```python
from build123d import *

# Parameters (mm, degrees)
EXTRUDE_1_DEPTH     = 6
EXTRUDE_2_DEPTH     = 4.2
SKETCH_3_R          = 2.35
EXTRUDE_3_DEPTH     = 2.8
SWEEP_START         = -2
SWEEP_1_DEPTH       = 4
CUT_EXTRUDE_1_DEPTH = 3


# Read off the part's stored shape, not the designer's step: По траектории1
with BuildPart() as part:
    # Эскиз1 → Бобышка-Вытянуть1 (new, symmetric)
    with BuildSketch(Plane(origin=(0, 0, 0), x_dir=(0, 0, -1), z_dir=(1, 0, 0))):
        Polygon((0, 0), (22, 0), (22, 19.3), (27, 19.3), (27, 21.8), (22, 21.8), (22, 26), (0, 26), (0, 21.8), (-5, 21.8), (-5, 19.3), (0, 19.3), align=None)
    extrude(amount=EXTRUDE_1_DEPTH, both=True)

    # Эскиз2 → Бобышка-Вытянуть2 (add)
    with BuildSketch(Plane(origin=(0, 26, 0), x_dir=(1, 0, 0), z_dir=(0, 1, 0))):
        with BuildLine():
            Line((-2.75, 12), (-2.75, 11.332682252))
            ThreePointArc((-2.75, 11.332682252), (0, 0), (2.75, 11.332682252))
            Line((2.75, 11.332682252), (2.75, 12))
            ThreePointArc((2.75, 12), (0, 14.75), (-2.75, 12))
        make_face()
    extrude(amount=EXTRUDE_2_DEPTH)

    # Эскиз3 → Бобышка-Вытянуть3 (add)
    with BuildSketch(Plane(origin=(0, 30.2, 0), x_dir=(1, 0, 0), z_dir=(0, 1, 0))):
        with Locations(Location((0, 6, 0), (0, 0, 270))):
            Circle(SKETCH_3_R)
    extrude(amount=EXTRUDE_3_DEPTH)

    # По траектории1 outline → По траектории1 (add)
    with BuildSketch(Plane.YZ.offset(SWEEP_START)):
        with BuildLine():
            Line((7.5, -22), (5, -22))
            add(Edge.make_bspline(
                [(5, -22), (5.069741994, -22.788251561), (5.125958635, -24.404153677), (4.878573381, -26.772120173), (4.395772619, -28.378294328), (3.83166606, -29.588406839), (3.21879889, -30.61604033), (2.403361035, -31.959681467), (1.936450048, -33.447187834), (1.879246473, -34.586937516), (2.09656871, -35.628227488), (2.472597261, -36.523725644), (2.84782964, -37.107918611), (3.067609014, -37.407797225)],
                knots=[0, 0, 0, 0, 0.166666667, 0.333333333, 0.5, 0.534253468, 0.625, 0.75, 0.8125, 0.875, 0.916666667, 0.958333333, 1, 1, 1, 1], degree=3))
            Line((3.067609014, -37.407797225), (5.173227765, -36.060069628))
            add(Edge.make_bspline(
                [(7.5, -22), (7.567173372, -22.882492449), (7.618252767, -24.686876341), (7.299304344, -27.455245749), (6.663696491, -29.460064755), (5.924563706, -30.955136787), (5.18985295, -32.152025941), (4.582294135, -33.24339685), (4.389602767, -34.062522123), (4.406362916, -34.546823904), (4.535371286, -35.013924669), (4.759350216, -35.482390845), (5.013826459, -35.862321947), (5.173227765, -36.060069628)],
                knots=[0, 0, 0, 0, 0.166666667, 0.333333333, 0.5, 0.534253468, 0.625, 0.75, 0.8125, 0.875, 0.916666667, 0.958333333, 1, 1, 1, 1], degree=3))
        make_face()
    extrude(amount=SWEEP_1_DEPTH)

    # Эскиз6 → Вырез-Вытянуть1 (cut)
    with BuildSketch(Plane(origin=(0, 21.8, 0), x_dir=(1, 0, 0), z_dir=(0, 1, 0))):
        with BuildLine():
            Line((-0.5, 27), (-0.5, 25.645643924))
            ThreePointArc((-0.5, 25.645643924), (0, 23.25), (0.5, 25.645643924))
            Line((0.5, 25.645643924), (0.5, 27))
            Line((0.5, 27), (0, 27))
            Line((0, 27), (-0.5, 27))
        make_face()
        with BuildLine():
            Line((0.5, -5), (0.5, -3.645643924))
            ThreePointArc((0.5, -3.645643924), (0, -1.25), (-0.5, -3.645643924))
            Line((-0.5, -3.645643924), (-0.5, -5))
            Line((-0.5, -5), (0, -5))
            Line((0, -5), (0.5, -5))
        make_face()
    extrude(amount=-CUT_EXTRUDE_1_DEPTH, mode=Mode.SUBTRACT)


solid = part.part
```
Part model, mm, in its own coordinate system. A direction names the side the tool comes from. Give positions to 0.01 mm unless a question says otherwise; leave off trailing zeros. Write each loop counter-clockwise with the first axis right and the second up, starting at its lowest first coordinate (ties: lowest second). Pieces come first, ordered by that corner, then holes. Notation, with made-up numbers: (13, -33) -> (20, -33) arc R9 cw to (20, -26) -> close; hole circle Ø6 at (21.5, 60). An arc over 180 degrees is marked (long way). Put each result on its own line as item: value. Start each with the question number.
Item 1: Cut at C-C (z = -24.5). State how many separate pieces and enclosed holes the cut face has, then the cut area to 3 significant figures.
Item 2: Which spindle directions (+Z, -Z, +X, -X, +Y, -Y) get a long thin tool onto all of the face, cutting with end or side? Do faces 5 (the face through (-0.5, 21, 4)), 6 (the face through (1.42, 21.8, -24.54)), 7 (the face through (1.42, 21.8, 2.47)). Say none if no direction does.
Item 3: Cut at A-A (z = 2.5). List the corners of the cut face in (x, y), then the cut area to 4 significant figures.
Item 4: Cut at D-D (y = 17.5). List the corners of the cut face in (x, z), then the cut area to 3 significant figures.
Item 5: Wall check: L1, parallel to X at y = 20.15, z = -24.5; L2, parallel to Y at x = 5.25, z = -2; L3, parallel to Y at x = 3, z = 1.5. Give the ranges that are in metal, low to high. Write a range as [from, to].
Item 6: Cut at B-B (x = -4.25). List the corners of the cut face in (y, z).
Item 7: Pin check, flat tips, straight feed: pin 1 Ø3 at (x, z) = (-1.5, -2) entering from +Y; pin 2 Ø3 at (x, z) = (-1, -31.5) entering from +Y; pin 3 Ø5.5 at (x, z) = (-2, -23.5) entering from +Y. Stop position of each tip, or through.
Item 8: Pull direction X, two halves, no side cores. Call faces 1 (the face through (0, 26, -16)), 2 (the face through (2, 5, -30)), 3 (the face through (0.06, 28.07, -14.75)), 4 (the face through (-0.05, 20.57, -23.25)): pulls with the +X half, pulls with the -X half, needs draft (parallel to the pull), parting line crosses it, or undercut.
Answer list:
1. separate pieces: 3
1. enclosed holes: 0
1. area: 33.7 mm2
2. face 5: +Z, +Y, -Y
2. face 6: -Z, +X, -X, +Y
2. face 7: +Z, +X, -X, +Y
3. outline: (-6, 19.3) -> (-1.25, 19.3) -> (-1.25, 21.8) -> (-6, 21.8) -> close; (1.25, 19.3) -> (6, 19.3) -> (6, 21.8) -> (1.25, 21.8) -> close
3. area: 23.75 mm2
4. outline: (-6, -22) -> (6, -22) -> (6, 0) -> (-6, 0) -> close
4. area: 264 mm2
5. L1: x = [-6, -1.25], [1.25, 6]
5. L2: y = [0, 26]
5. L3: y = [19.3, 21.8]
6. outline: (0, -22) -> (19.3, -22) -> (19.3, -27) -> (21.8, -27) -> (21.8, -22) -> (26, -22) -> (26, -10.24) -> (30.2, -10.24) -> (30.2, -1.76) -> (26, -1.76) -> (26, 0) -> (21.8, 0) -> (21.8, 5) -> (19.3, 5) -> (19.3, 0) -> (0, 0) -> close
7. pin 1: stops at y = 30.2
7. pin 2: stops at y = 6.39
7. pin 3: stops at y = 26
8. face 1: needs draft
8. face 2: pulls with the +X half
8. face 3: parting line crosses it
8. face 4: undercut
